Geometry check sheet. Reference: the model listing, model coordinates, mm. A direction names the side the tool comes from. Coordinates: 2 decimals unless noted, no trailing zeros. Write each loop counter-clockwise with the first axis right and the second up, starting at its lowest first coordinate (ties: lowest second). Pieces come first, ordered by that corner, then holes. Notation, with made-up numbers: (5.25, 40) -> (19.25, 40) arc R14 cw to (19.25, 52) -> close; hole circle Ø1 at (-4, 88). An arc over 180 degrees is marked (long way). Use a Markdown table: item, result.
```python
from build123d import *

# Parameters (mm, degrees)
F0_W           = 51.2
F0_H           = 22
F1_DEPTH       = 6
F2_R           = 2.1
F3_DEPTH       = 6.001
F5_DEPTH       = 6.001
F8_DEPTH       = 13.5
F9_W           = 14.7
F9_H           = 10
F10_DEPTH      = 12.001
F11_T1_DEPTH   = 6
F12_R          = 1.6
F13_DEPTH      = 34.601
F13_DEPTH_BACK = 16.601
F14_R          = 2.75
F15_DEPTH      = 4.5
F15_DEPTH_BACK = 16.601
F17_DEPTH      = 4.5
F17_DEPTH_BACK = 25
F18_W          = 30
F18_H          = 17
F19_DEPTH      = 12.001
F20_T1_DEPTH   = 6
F20_T3_DEPTH   = 31
F20_T5_DEPTH   = 22.6993813232


# Not quite as in the source:
# - a fillet or chamfer that OpenCascade refuses, or shapes differently, is made with other operations: its cross-section is extruded or revolved along the edge and cut away or added


with BuildPart() as f1:
    # F0 (on Top) → F1 (new body)
    with BuildSketch(Plane.XY):
        Rectangle(F0_W, F0_H)
    extrude(amount=F1_DEPTH)

    # F2 (on face) → F3 (cut, through all)
    with BuildSketch(Plane.XY.offset(6)):
        with Locations((-20.5, 0)):
            Circle(F2_R)
        with Locations((20.5, 0)):
            Circle(F2_R)
    extrude(amount=-F3_DEPTH, mode=Mode.SUBTRACT)

    # F4 (on face) → F5 (cut, through all)
    with BuildSketch(Plane.XY.offset(6)):
        with BuildLine():
            Line((-1.5, 11), (-1.5, 0))
            ThreePointArc((-1.5, 0), (4.5, -6), (10.5, 0))
            Line((10.5, 0), (10.5, 11))
            Line((10.5, 11), (-1.5, 11))
        make_face()
    extrude(amount=-F5_DEPTH, mode=Mode.SUBTRACT)

    # F7 (on mid) → F8 (join, symmetric)
    with BuildSketch(Plane(origin=(4.5, 0, 0), x_dir=(0, -1, 0), z_dir=(-1, 0, 0))):
        Polygon((21, 6), (11, 6), (11, 0), (11, -6), (21, -6), align=None)
    extrude(amount=F8_DEPTH, both=True)

    # F9 (on face) → F10 (cut, through all)
    with BuildSketch(Plane(origin=(0, 0, -6), x_dir=(1, 0, 0), z_dir=(0, 0, -1))):
        with Locations((4.5, 16)):
            Rectangle(F9_W, F9_H)
    extrude(amount=-F10_DEPTH, mode=Mode.SUBTRACT)

    # F11: fillet of radius 10 on 2 edges, made by hand

    # F11_s2 → F11_t1 (join)
    with BuildSketch(Plane.XY):
        with BuildLine():
            ThreePointArc((-19, -11), (-11.9289321881, -13.9289321881), (-9, -21))
            Line((-9, -21), (-9, -11))
            Line((-9, -11), (-19, -11))
        make_face()
        with BuildLine():
            ThreePointArc((25.6, -11), (20.125992126, -14.5433148766), (18, -20.7077288796))
            Line((18, -20.7077288796), (18, -11))
            Line((18, -11), (25.6, -11))
        make_face()
    extrude(amount=F11_T1_DEPTH)

    # F12 (on face) → F13 (cut, two sides)
    with BuildSketch(Plane(origin=(-9, 0, 0), x_dir=(0, -1, 0), z_dir=(-1, 0, 0))) as f13_sk:
        with Locations((16, -1)):
            Circle(F12_R)
    extrude(amount=-F13_DEPTH, mode=Mode.SUBTRACT)
    extrude(f13_sk.sketch, amount=F13_DEPTH_BACK, mode=Mode.SUBTRACT)

    # F14 (on face) → F15 (cut, two sides)
    with BuildSketch(Plane(origin=(-9, 0, 0), x_dir=(0, -1, 0), z_dir=(-1, 0, 0))) as f15_sk:
        with Locations((16, -1)):
            Circle(F14_R)
    extrude(amount=-F15_DEPTH, mode=Mode.SUBTRACT)
    extrude(f15_sk.sketch, amount=F15_DEPTH_BACK, mode=Mode.SUBTRACT)

    # F16 (on face) → F17 (cut, two sides)
    with BuildSketch(Plane.YZ.offset(18)) as f17_sk:
        Polygon((-14.3545517328, -3.85), (-12.7091034656, -1), (-14.3545517328, 1.85), (-17.6454482672, 1.85), (-19.2908965344, -1), (-17.6454482672, -3.85), align=None)
    extrude(amount=-F17_DEPTH, mode=Mode.SUBTRACT)
    extrude(f17_sk.sketch, amount=F17_DEPTH_BACK, mode=Mode.SUBTRACT)

    # F18 (on face) → F19 (cut, through all)
    with BuildSketch(Plane.XY.offset(6)):
        with Locations((0, 2.5)):
            Rectangle(F18_W, F18_H)
    extrude(amount=-F19_DEPTH, mode=Mode.SUBTRACT)

    # F20: fillet of radius 5 on 9 edges, made by hand

    # F20_s2 → F20_t1 (join)
    with BuildSketch(Plane.XY):
        with BuildLine():
            ThreePointArc((-15, -1), (-13.5355339059, -4.5355339059), (-10, -6))
            Line((-10, -6), (-15, -6))
            Line((-15, -6), (-15, -1))
        make_face()
        with BuildLine():
            ThreePointArc((10, -6), (13.5355339059, -4.5355339059), (15, -1))
            Line((15, -1), (15, -6))
            Line((15, -6), (10, -6))
        make_face()
    extrude(amount=F20_T1_DEPTH)

    # F20_s4 → F20_t3 (cut)
    with BuildSketch(Plane.XY.offset(-12.5)):
        with BuildLine():
            ThreePointArc((-25.6, -6), (-24.1355339059, -9.5355339059), (-20.6, -11))
            Line((-20.6, -11), (-25.6, -11))
            Line((-25.6, -11), (-25.6, -6))
        make_face()
        with BuildLine():
            ThreePointArc((25.6, 6), (24.1355339059, 9.5355339059), (20.6, 11))
            Line((20.6, 11), (25.6, 11))
            Line((25.6, 11), (25.6, 6))
        make_face()
        with BuildLine():
            ThreePointArc((20, 11), (16.4644660941, 9.5355339059), (15, 6))
            Line((15, 6), (15, 11))
            Line((15, 11), (20, 11))
        make_face()
        with BuildLine():
            ThreePointArc((-20.6, 11), (-24.1355339059, 9.5355339059), (-25.6, 6))
            Line((-25.6, 6), (-25.6, 11))
            Line((-25.6, 11), (-20.6, 11))
        make_face()
        with BuildLine():
            ThreePointArc((-15, 6), (-16.4644660941, 9.5355339059), (-20, 11))
            Line((-20, 11), (-15, 11))
            Line((-15, 11), (-15, 6))
        make_face()
    extrude(amount=F20_T3_DEPTH, mode=Mode.SUBTRACT)

    # F20_s6 → F20_t5 (cut)
    with BuildSketch(Plane.XY.offset(-8.3496906616)):
        with BuildLine():
            ThreePointArc((25.6, -7.6601237354), (24.9204937989, -10.1767352138), (23.0666666667, -12.0093254501))
            ThreePointArc((23.0666666667, -12.0093254501), (24.298766569, -11.4179026654), (25.6, -11))
            Line((25.6, -11), (25.6, -7.6601237354))
        make_face()
    extrude(amount=F20_T5_DEPTH, mode=Mode.SUBTRACT)


solid = f1.part
```
Item 1: Depth check by flat-ended pin: P1, Ø5.5, axis at x = 20.5, y = 0, coming from the -Z side; P2, Ø10, axis at x = -6.5, y = -5.5, coming from the +Z side; P3, Ø0.8, axis at x = -19.5, z = 2, coming from the -Y side; P4, Ø3, axis at y = -16, z = -0.5, coming from the -X side. Enter the tip coordinate at first touch or a pass-through.
Answer block:
| item | result |
|---|---|
| P1 | stops at z = 0 |
| P2 | stops at z = 6 |
| P3 | stops at y = -11 |
| P4 | stops at x = -4.5 |
Item 2: Section check A-A on y = 0. Record the boundary of the cut face in (x, z).
Answer block:
| item | result |
|---|---|
| outline | (-25.6, 0) -> (-22.6, 0) -> (-22.6, 6) -> (-25.6, 6) -> close; (-18.4, 0) -> (-15, 0) -> (-15, 6) -> (-18.4, 6) -> close; (15, 0) -> (18.4, 0) -> (18.4, 6) -> (15, 6) -> close; (22.6, 0) -> (25.6, 0) -> (25.6, 6) -> (22.6, 6) -> close |
Item 3: Section check D-D on z = -0.5. Record the boundary of the cut face in (x, y).
Answer block:
| item | result |
|---|---|
| outline | (-9, -21) -> (-2.85, -21) -> (-2.85, -17.52) -> (-4.5, -17.52) -> (-4.5, -18.7) -> (-9, -18.7) -> close; (-9, -13.3) -> (-4.5, -13.3) -> (-4.5, -14.48) -> (-2.85, -14.48) -> (-2.85, -11) -> (-9, -11) -> close; (11.85, -21) -> (18, -21) -> (18, -19) -> (13.5, -19) -> (13.5, -17.52) -> (11.85, -17.52) -> close; (11.85, -14.48) -> (13.5, -14.48) -> (13.5, -13) -> (18, -13) -> (18, -11) -> (11.85, -11) -> close |
Item 4: Section check B-B on y = 3.5. Record the boundary of the cut face in (x, z), then the cut area to 3 significant figures.
Answer block:
| item | result |
|---|---|
| outline | (-25.6, 0) -> (-15, 0) -> (-15, 6) -> (-25.6, 6) -> close; (15, 0) -> (25.6, 0) -> (25.6, 6) -> (15, 6) -> close |
| area | 127 mm^2 |
Item 5: Section check C-C on z = 4.75. Record the boundary of the cut face in (x, y), then the cut area to 3 significant figures.
Answer block:
| item | result |
|---|---|
| outline | (-25.6, -6) arc R5 ccw to (-20.6, -11) -> (-19, -11) arc R10 cw to (-9, -21) -> (-2.85, -21) -> (-2.85, -11) -> (11.85, -11) -> (11.85, -21) -> (18, -21) -> (18, -20.71) arc R10 cw to (23.07, -12.01) arc R5 ccw to (25.6, -7.66) -> (25.6, 6) arc R5 ccw to (20.6, 11) -> (20, 11) arc R5 ccw to (15, 6) -> (15, -1) arc R5 cw to (10, -6) -> (-10, -6) arc R5 cw to (-15, -1) -> (-15, 6) arc R5 ccw to (-20, 11) -> (-20.6, 11) arc R5 ccw to (-25.6, 6) -> close; hole circle Ø4.2 at (-20.5, 0); hole circle Ø4.2 at (20.5, 0) |
| area | 734 mm^2 |
Item 6: Tool access check on faces 1 (the cylindrical face through (13, -5, 3)), 2 (the flat face through (-4.5, -18, -1)), 3 (the flat face through (-2.85, -16, 1)). Record the directions out of +Z, -Z, +X, -X, +Y, -Y that give a thin tool (end or side, any length) a straight path to the whole face; none if there is none.
Answer block:
| item | result |
|---|---|
| face 1 | +Z, -Z, +Y |
| face 2 | -X |
| face 3 | +Z, -Z, -Y |
Item 7: Mould release check, pull along X, two halves, no side actions. Record for faces 4 (the flat face through (-9, -16, -4)), 5 (the flat face through (11.85, -16, 1)), 6 (the flat face through (0.4, -6.5, 0)), 7 (the cylindrical face through (24.94, -10.14, 2.96)): +X half, -X half, draft (parallel to the pull), parting line (faces both ways), or undercut.
Answer block:
| item | result |
|---|---|
| face 4 | -X half |
| face 5 | undercut |
| face 6 | draft |
| face 7 | +X half |
Item 8: Thickness scan on L1, parallel to X at y = 4, z = 3; L2, parallel to X at y = -1, z = 0.25; L3, parallel to Z at x = -6, y = -16. Record the ranges inside material, lowest first. Write a range as [from, to].
Answer block:
| item | result |
|---|---|
| L1 | x = [-25.6, -15], [15, 25.6] |
| L2 | x = [-25.6, -22.35], [-18.65, -15], [15, 18.65], [22.35, 25.6] |
| L3 | z = [-6, -3.75], [1.75, 6] |
